```python
from build123d import *

# Parameters (mm, degrees)
SKETCH1_W           = 40
SKETCH1_H           = 40
BOSS_EXTRUDE1_DEPTH = 40
CUT_EXTRUDE1_DEPTH  = 40
CUT_EXTRUDE2_DEPTH  = 40
CUT_EXTRUDE3_DEPTH  = 40
SKETCH5_W           = 20
SKETCH5_H           = 40
BOSS_EXTRUDE2_DEPTH = 20


with BuildPart() as part:
    # Sketch1 → Boss-Extrude1 (new body)
    with BuildSketch(Plane.XY):
        with Locations((20, 20)):
            Rectangle(SKETCH1_W, SKETCH1_H)
    extrude(amount=BOSS_EXTRUDE1_DEPTH)

    # Sketch2 → Cut-Extrude1 (cut)
    with BuildSketch(Plane.XY.offset(40)):
        Polygon((0, 20), (0, 40), (20, 40), align=None)
    extrude(amount=-CUT_EXTRUDE1_DEPTH, mode=Mode.SUBTRACT)

    # Sketch3 → Cut-Extrude2 (cut)
    with BuildSketch(Plane.ZY):
        Polygon((40, 0), (20, 20), (0, 40), (40, 40), align=None)
    extrude(amount=-CUT_EXTRUDE2_DEPTH, mode=Mode.SUBTRACT)

    # Sketch4 → Cut-Extrude3 (cut)
    with BuildSketch(Plane(origin=(0, 20, 20), x_dir=(1, 0, 0), z_dir=(0, 0.707106781, 0.707106781))):
        Polygon((0, 0), (20, -40), (0, -40), align=None)
    extrude(amount=-CUT_EXTRUDE3_DEPTH, mode=Mode.SUBTRACT)

    # Sketch5 → Boss-Extrude2 (add)
    with BuildSketch(Plane(origin=(40, 0, 0), x_dir=(0, 0, -1), z_dir=(1, 0, 0))):
        with Locations((-10, 20)):
            Rectangle(SKETCH5_W, SKETCH5_H)
    extrude(amount=-BOSS_EXTRUDE2_DEPTH)


solid = part.part
```
Can you work these out from the model? Positions are in its coordinate system, mm. A direction names the side the tool comes from. Round coordinates to 2 decimals unless told otherwise and drop trailing zeros. Loops run counter-clockwise (first coordinate to the right, second up) from the corner with the lowest first, then second, coordinate; pieces in that order, holes last. Notation, with made-up numbers: M 77.5,-27 L 91.5,-27 A19 ccw 91.5,7 Z; hole C -4,56.25 d5. An arc over 180 degrees is marked long. Answer as a JSON object with one key per item and string values. Group by question number.
Q1. Imagine slicing it at A-A, the plane y = 28. Please give me the cut outline in (x, z), then the cut area to 3 significant figures.
Q2. Will these pins go through, and if not, where does the flat tip stop? pin 1 (6 mm diameter, centred on x = 26.5, y = 25.5, fed in from +Z); pin 2 (6 mm diameter, centred on y = 30, z = 14.5, fed in from -X).
Q3. Please list where these lines run through material, in increasing order: L1, parallel to Z at x = 6.5, y = 20; L2, parallel to Z at x = 21, y = 17.5; L3, parallel to Y at x = 34.5, z = 28.5.
Q4. Imagine slicing it at B-B, the plane x = 27. Please give me the cut outline in (y, z), then the cut area to 3 significant figures.
Q5. Imagine slicing it at C-C, the plane z = 9. Please give me the cut outline in (x, y).
Q6. Imagine slicing it at D-D, the plane y = 23.5. Please give me the cut outline in (x, z), then the cut area to 3 significant figures.
Q7. On a 3-axis mill with a long thin cutter (end or side, diameter ignored), from which of +Z, -Z, +X, -X, +Y, -Y can I reach the whole of each face in a straight line? I mean faces 1 (the flat face through (20, 32, 12)), 2 (the flat face through (24, 0, 20)), 3 (the flat face through (30, 30, 20)). Say none if no direction works.
Findings:
{
 "1": {"outline": "M 8,0 L 40,0 L 40,20 L 20,20 L 20,12 L 8,12 Z", "area": "544 mm2"},
 "2": {"pin 1": "stops at z = 20", "pin 2": "stops at x = 20"},
 "3": {"L1": "z = 0 to 20", "L2": "z = 0 to 22.5", "L3": "y = 0 to 11.5"},
 "4": {"outline": "M 0,0 L 40,0 L 40,20 L 20,20 L 0,40 Z", "area": "1,000 mm2"},
 "5": {"outline": "M 0,9 L 3.18,0 L 40,0 L 40,40 L 20,40 L 20,31 L 11,31 L 0,20 Z"},
 "6": {"outline": "M 3.5,0 L 40,0 L 40,20 L 20,20 L 20,16.5 L 3.5,16.5 Z", "area": "672 mm2"},
 "7": {"face 1": "+Z, -X, +Y", "face 2": "+Z, -Z, +X, -X, -Y", "face 3": "+Z, +X, -X, +Y"}
}
